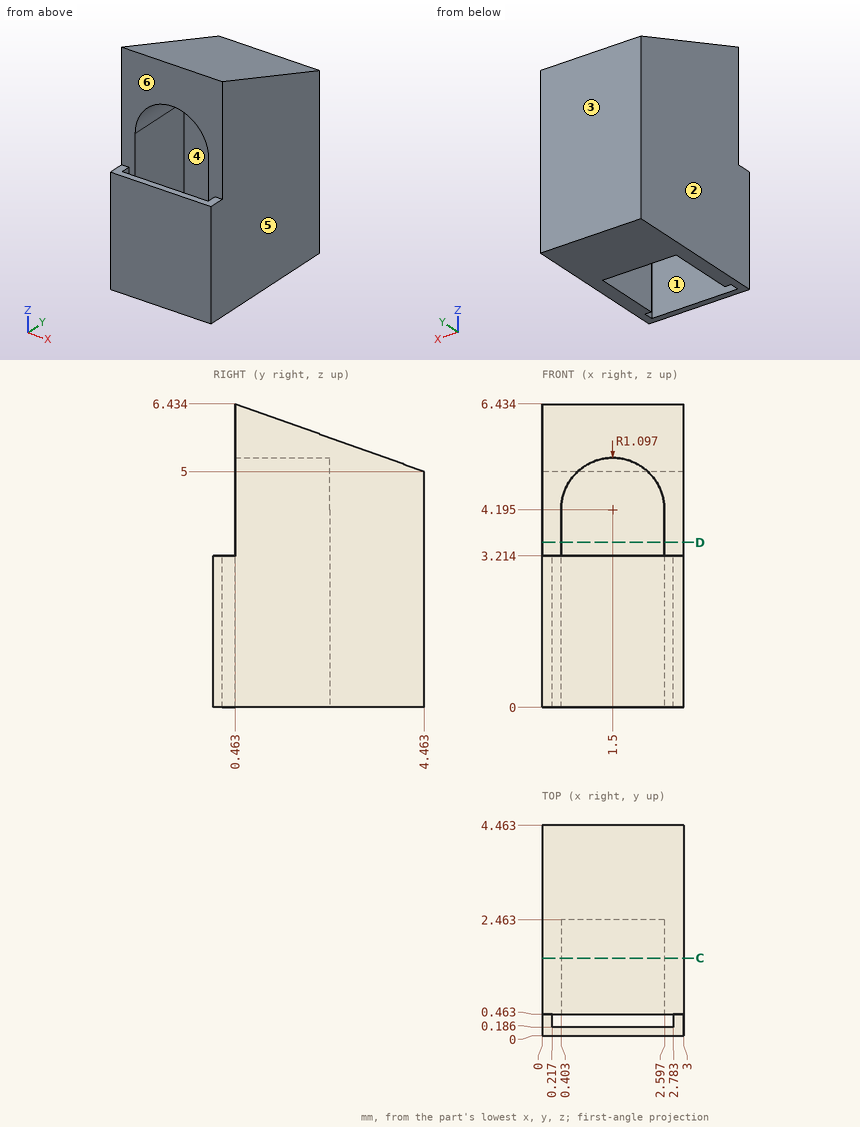
Design review of the part shown in the three views and the two pictorial views. Dimensions are in mm from the part's minimum x, y and z. A direction names the side the tool comes from. Round coordinates to 2 decimals unless told otherwise and drop trailing zeros. Write each loop counter-clockwise with the first axis right and the second up, starting at its lowest first coordinate (ties: lowest second). Pieces come first, ordered by that corner, then holes. Notation, with made-up numbers: (82, -19.5) -> (119, -19.5) arc R20 ccw to (119, -6.5) -> close; hole circle Ø3 at (54, 37.5). An arc over 180 degrees is marked (long way). One line per question, with ' | ' between items. Start each with the question number.
1) Wall thickness on line 1 along X through (y, z) = (1.25, 0.5); line 2 along Y through (x, z) = (2.65, 1) (1 decimal); line 3 along X through (y, z) = (0.4, 2.5): over which ranges is each line inside the solid? List them lowest first.
2) Add section C-C (y = 1.65). Write out the cut boundary in (x, z) (1 decimal).
3) Mouldability with a two-part tool opening along X and no side actions: class the marked faces 1, 2 and 3 as +X half, -X half, draft (parallel to the pull), parting line (faces both ways), or undercut.
4) For pin 1 Ø0.9 at (x, z) = (1.5, 4.5) entering from -Y, flat-tipped, find the tip position at first contact; note if it passes through.
5) Machinability: for the marked faces 4, 5 and 6, which of the approach directions +Z, -Z, +X, -X, +Y, -Y give a long, thin tool a straight path to every point of the face, cutting with its end or side? Answer none if there is none.
6) Add section D-D (z = 3.5). Write out the cut boundary in (x, y).
Reported:
1) line 1: x = 0 to 0.4, 2.6 to 3 | line 2: y = 0 to 0.2, 0.5 to 4.5 | line 3: x = 0 to 0.22, 2.78 to 3
2) outline: (0, 0) -> (0.4, 0) -> (0.4, 4.2) arc R1.1 cw to (2.6, 4.2) -> (2.6, 0) -> (3, 0) -> (3, 6) -> (0, 6) -> close
3) face 1: undercut | face 2: -X half | face 3: draft
4) pin 1: stops at y = 2.46
5) face 4: -Z | face 5: +Z, -Z, +X, +Y, -Y | face 6: +Z
6) outline: (0, 0.46) -> (0.4, 0.46) -> (0.4, 2.46) -> (2.6, 2.46) -> (2.6, 0.46) -> (3, 0.46) -> (3, 4.46) -> (0, 4.46) -> close
